from build123d import *

# Parameters (mm, degrees)
SKETCH_1_W          = 40
SKETCH_1_H          = 40
SKETCH_1_R          = 1.5
EXTRUDE_1_DEPTH     = 10
FILLET_1_R          = 2
SKETCH_2_R          = 3
CUT_EXTRUDE_1_DEPTH = 4


with BuildPart() as part:
    # Эскиз1 → Бобышка-Вытянуть1 (new body)
    with BuildSketch(Plane(origin=(0, 0, 0), x_dir=(1, 0, 0), z_dir=(0, 1, 0))):
        with Locations((0.283687943, -8.156028369)):
            Rectangle(SKETCH_1_W, SKETCH_1_H)
        with Locations(Location((-15.716312057, 7.843971631, 0), (0, 0, 270))):
            Circle(SKETCH_1_R, mode=Mode.SUBTRACT)
        with Locations(Location((16.283687943, 7.843971631, 0), (0, 0, 270))):
            Circle(SKETCH_1_R, mode=Mode.SUBTRACT)
        with Locations(Location((16.283687943, -24.156028369, 0), (0, 0, 270))):
            Circle(SKETCH_1_R, mode=Mode.SUBTRACT)
        with Locations(Location((-15.716312057, -24.156028369, 0), (0, 0, 270))):
            Circle(SKETCH_1_R, mode=Mode.SUBTRACT)
    extrude(amount=EXTRUDE_1_DEPTH)

    # Скругление1
    fillet_1_edges = [part.edges().sort_by_distance(p)[0] for p in [
        (-19.716312057, 5, -11.843971631),
        (20.283687943, 5, -11.843971631),
        (20.283687943, 5, 28.156028369),
        (-19.716312057, 5, 28.156028369),
    ]]
    fillet(fillet_1_edges, radius=FILLET_1_R)

    # Эскиз2 → Вырез-Вытянуть1 (cut)
    with BuildSketch(Plane(origin=(0, 10, 0), x_dir=(1, 0, 0), z_dir=(0, 1, 0))):
        with Locations(Location((-15.716312057, 7.843971631, 0), (0, 0, 270))):
            Circle(SKETCH_2_R)
        with Locations(Location((16.283687943, 7.843971631, 0), (0, 0, 270))):
            Circle(SKETCH_2_R)
        with Locations(Location((16.283687943, -24.156028369, 0), (0, 0, 270))):
            Circle(SKETCH_2_R)
        with Locations(Location((-15.716312057, -24.156028369, 0), (0, 0, 270))):
            Circle(SKETCH_2_R)
    extrude(amount=-CUT_EXTRUDE_1_DEPTH, mode=Mode.SUBTRACT)


solid = part.part
Geometry: final body of the model. Coordinates: model frame, mm. A direction names the side the tool comes from. Coordinates: 2 decimals unless noted, no trailing zeros. Order: outer loops, then holes, each group sorted by start corner. A loop starts at its lowest first (then second) coordinate and runs counter-clockwise, first axis right, second up. Notation, with made-up numbers: M 79,36.5 L 91,36.5 A8 cw 91,42.5 Z; hole C 3.5,-27.75 d3. An arc over 180 degrees is marked long. One line per question, with ' | ' between items. Start each with the question number.
Item 1: Cut plane C-C, the plane x = 17. Return the cut outline in (y, z).
Item 2: Ray query, probe 1 along X at (y, z) = (7.75, -6); probe 2 along Z at (x, y) = (-16, 3); probe 3 along X at (y, z) = (7.5, -7). Return the intervals inside material, ascending. Write a range as [from, to].
Item 3: Cut plane A-A, the plane z = 25. Return the cut outline in (x, y), then the cut area to 3 significant figures.
Item 4: Draft query along Z for faces 1 (the cylindrical face through (-19.15, 5.07, -11.24)), 2 (the cylindrical face through (19.68, 5.07, 27.59)), 3 (the flat face through (-14, 6, -7)). Return one class per face: released by +Z, released by -Z, zero draft, split by the parting line, or undercut.
Item 5: Cut plane B-B, the plane y = 3. Return the cut outline in (x, z).
Item 6: Pin query (flat end, axial travel): pin 1 Ø1.8 at (x, z) = (-15.72, 24.16) entering from +Y; pin 2 Ø4 at (x, z) = (16.28, 24.16) entering from +Y. Return the tip coordinate at first contact, or that it passes through.
Item 7: Set-up query: faces 4 (the cylindrical face through (17.18, 8.03, 27.02)), 5 (the flat face through (0, 0, 8)). Return all of +Z, -Z, +X, -X, +Y, -Y with unobstructed straight access to the full face (end or side cutting, diameter ignored); none if empty.
A:
1) outline: M 0,-11.84 L 10,-11.84 L 10,-10.76 L 6,-10.76 L 6,-9.16 L 0,-9.16 Z; M 0,-6.53 L 6,-6.53 L 6,-4.93 L 10,-4.93 L 10,21.24 L 6,21.24 L 6,22.84 L 0,22.84 Z; M 0,25.47 L 6,25.47 L 6,27.07 L 10,27.07 L 10,28.16 L 0,28.16 Z
2) probe 1: x = [-19.72, -18.08], [-13.35, 13.92], [18.65, 20.28] | probe 2: z = [-11.84, -9.32], [-6.37, 22.68], [25.63, 28.16] | probe 3: x = [-19.72, -18.6], [-12.84, 13.4], [19.16, 20.28]
3) outline: M -19.72,0 L -16.96,0 L -16.96,6 L -18.6,6 L -18.6,10 L -19.72,10 Z; M -14.48,0 L 15.04,0 L 15.04,6 L 13.4,6 L 13.4,10 L -12.84,10 L -12.84,6 L -14.48,6 Z; M 17.52,0 L 20.28,0 L 20.28,10 L 19.16,10 L 19.16,6 L 17.52,6 Z | area: 324 mm2
4) face 1: released by -Z | face 2: released by +Z | face 3: undercut
5) outline: M -19.72,-9.84 A2 ccw -17.72,-11.84 L 18.28,-11.84 A2 ccw 20.28,-9.84 L 20.28,26.16 A2 ccw 18.28,28.16 L -17.72,28.16 A2 ccw -19.72,26.16 Z; hole C -15.72,-7.84 d3; hole C -15.72,24.16 d3; hole C 16.28,-7.84 d3; hole C 16.28,24.16 d3
6) pin 1: passes through | pin 2: stops at y = 6
7) face 4: +Y | face 5: +Z, -Z, +X, -X, -Y
